CAD build for the part. Positions are in the model's coordinates, mm. A direction names the side the tool comes from. Round coordinates to 2 decimals unless told otherwise and drop trailing zeros. Write each loop counter-clockwise with the first axis right and the second up, starting at its lowest first coordinate (ties: lowest second). Pieces come first, ordered by that corner, then holes. Notation, with made-up numbers: (32.5, -6) - (78.5, -6) arc R14 cw to (78.5, -2) - close; hole circle Ø2 at (-15, -3). An arc over 180 degrees is marked (long way). Answer in a Markdown table with one row per item.
```python
from build123d import *

# Parameters (mm, degrees)
DIE_DEPTH                                      = 19.05
DRILL_CBORE_FOR_1_4_SHCS_SHALLOW_1_D           = 7.1374
DRILL_CBORE_FOR_1_4_SHCS_SHALLOW_1_CBORE_D     = 10.3124
DRILL_CBORE_FOR_1_4_SHCS_SHALLOW_1_CBORE_DEPTH = 7.112


with BuildPart() as part:
    # Sketch1 → Die (new body)
    with BuildSketch(Plane.XY):
        with BuildLine():
            Line((-81.026, 63.5), (-7.874, 63.5))
            ThreePointArc((-7.874, 63.5), (-2.306241205, 61.193758795), (0, 55.626))
            Line((0, 55.626), (0, 7.874))
            ThreePointArc((0, 7.874), (-2.306241205, 2.306241205), (-7.874, 0))
            Line((-7.874, 0), (-81.026, 0))
            ThreePointArc((-81.026, 0), (-86.593758795, 2.306241205), (-88.9, 7.874))
            Line((-88.9, 7.874), (-88.9, 55.626))
            ThreePointArc((-88.9, 55.626), (-86.593758795, 61.193758795), (-81.026, 63.5))
        make_face()
    extrude(amount=DIE_DEPTH)

    # Drill&CBore For 1/4 SHCS (Shallow)1 (through all)
    with Locations(Plane.XY.offset(19.05)):
        with Locations((-10.414, 12.192), (-78.74, 52.578)):
            CounterBoreHole(DRILL_CBORE_FOR_1_4_SHCS_SHALLOW_1_D / 2, DRILL_CBORE_FOR_1_4_SHCS_SHALLOW_1_CBORE_D / 2, DRILL_CBORE_FOR_1_4_SHCS_SHALLOW_1_CBORE_DEPTH)


solid = part.part
```
Q1. Flat gauge pin, fed straight in: pin 1 (3 mm diameter, centred on x = -12, y = 11, fed in from +Z). Where does the tip first touch, or does it go through?
Computed:
| item | result |
|---|---|
| pin 1 | passes through |
Q2. Saw through at B-B on z = 16. List the corners of the cut face in (x, y), then the cut area to 3 significant figures.
Computed:
| item | result |
|---|---|
| outline | (-88.9, 7.87) arc R7.87 ccw to (-81.03, 0) - (-7.87, 0) arc R7.87 ccw to (0, 7.87) - (0, 55.63) arc R7.87 ccw to (-7.87, 63.5) - (-81.03, 63.5) arc R7.87 ccw to (-88.9, 55.63) - close; hole circle Ø10.31 at (-78.74, 52.58); hole circle Ø10.31 at (-10.41, 12.19) |
| area | 5,420 mm2 |
Q3. 3-axis set-ups, long thin cutter, end or side, ignore diameter. For faces 1 (the flat face through (-45, 63.5, 9)), 2 (the flat face through (-80, 49, 11.938)): which of +Z, -Z, +X, -X, +Y, -Y reach the whole face in a straight line?
Computed:
| item | result |
|---|---|
| face 1 | +Z, -Z, +X, -X, +Y |
| face 2 | +Z |
Q4. Pull direction X, two halves, no side cores. Call faces 3 (the flat face through (-44, 32, 19.05)), 4 (the cylindrical face through (-86.655, 61.132, 9.392)), 5 (the flat face through (-14, 11, 11.938)): released by +X, released by -X, zero draft, split by the parting line, or undercut.
Computed:
| item | result |
|---|---|
| face 3 | zero draft |
| face 4 | released by -X |
| face 5 | undercut |
Q5. Saw through at C-C on z = 2. List the corners of the cut face in (x, y), then the cut area to 3 significant figures.
Computed:
| item | result |
|---|---|
| outline | (-88.9, 7.87) arc R7.87 ccw to (-81.03, 0) - (-7.87, 0) arc R7.87 ccw to (0, 7.87) - (0, 55.63) arc R7.87 ccw to (-7.87, 63.5) - (-81.03, 63.5) arc R7.87 ccw to (-88.9, 55.63) - close; hole circle Ø7.14 at (-78.74, 52.58); hole circle Ø7.14 at (-10.41, 12.19) |
| area | 5,510 mm2 |
Q6. Drill centre lines: line 1 (Y direction, x = -78.5, z = 14.5); line 2 (X direction, y = 15, z = 17.5); line 3 (Y direction, x = -75.5, z = 17.5). Where is each one in solid material? Low to high.
Computed:
| item | result |
|---|---|
| line 1 | y = 0 to 47.43, 57.73 to 63.5 |
| line 2 | x = -88.9 to -14.74, -6.09 to 0 |
| line 3 | y = 0 to 48.57, 56.59 to 63.5 |
Q7. Saw through at A-A on x = -78.74. List the corners of the cut face in (y, z).
Computed:
| item | result |
|---|---|
| outline | (0, 0) - (49.01, 0) - (49.01, 11.94) - (47.42, 11.94) - (47.42, 19.05) - (0, 19.05) - close; (56.15, 0) - (63.5, 0) - (63.5, 19.05) - (57.73, 19.05) - (57.73, 11.94) - (56.15, 11.94) - close |
